Here's how the part is built. I have some questions about the finished solid (model axes, mm). A direction names the side the tool comes from. Round coordinates to 2 decimals unless told otherwise and drop trailing zeros. Loops run counter-clockwise (first coordinate to the right, second up) from the corner with the lowest first, then second, coordinate; pieces in that order, holes last. Notation, with made-up numbers: M -4.5,-27.5 L 17.5,-27.5 A20 cw 17.5,-5.5 Z; hole C 81,82 d5. An arc over 180 degrees is marked long. Put each result on its own line as item: value. Start each with the question number.
```python
from build123d import *

# Parameters (mm, degrees)
SKETCH_3_R           = 9.5
CUT_EXTRUDE_1_DEPTH  = 321.526909947
SKETCH_4_R           = 9.5
CUT_EXTRUDE_2_DEPTH  = 321.526909947
SKETCH_5_R           = 9.5
CUT_EXTRUDE_3_DEPTH  = 321.526909947
SKETCH_6_R           = 9.5
CUT_EXTRUDE_4_DEPTH  = 321.526909947
SKETCH_7_R           = 9.5
CUT_EXTRUDE_5_DEPTH  = 321.526909947
SKETCH_8_R           = 9.5
CUT_EXTRUDE_6_DEPTH  = 321.526909947
SKETCH_9_R           = 9.5
CUT_EXTRUDE_7_DEPTH  = 321.526909947
SKETCH_10_R          = 9.5
CUT_EXTRUDE_8_DEPTH  = 321.526909947
SKETCH_11_R          = 9.5
CUT_EXTRUDE_9_DEPTH  = 321.526909947
SKETCH_12_R          = 9.5
CUT_EXTRUDE_10_DEPTH = 321.526909947
SKETCH_13_R          = 9.5
CUT_EXTRUDE_11_DEPTH = 321.526909947
SKETCH_14_R          = 9.5
CUT_EXTRUDE_12_DEPTH = 321.526909947


with BuildPart() as part:
    # Эскиз1 → Повернуть1 (revolve)
    with BuildSketch(Plane.XY, mode=Mode.PRIVATE) as revolve_1_sk:
        Polygon((0, 0), (265, 0), (265, 127.5), (239, 127.5), (239, 100), (239, 95), (220, 95), (220, 94), (200, 94), (144, 65.5), (70, 65.5), (25, 41), (3, 41), (3, 45), (0, 45), align=None)
    revolve(revolve_1_sk.sketch.rotate(Axis((0, 0, 0), (1, 0, 0)), 90), axis=Axis((0, 0, 0), (1, 0, 0)))

    # Эскиз2 → Вырез-Повернуть1 (revolve, cut)
    with BuildSketch(Plane.XY, mode=Mode.PRIVATE) as cut_revolve_1_sk:
        with BuildLine():
            Line((0, 0), (257, 0))
            Line((257, 0), (257, 34))
            Line((257, 34), (239, 34))
            Line((239, 34), (239, 47))
            Line((239, 47), (220, 47))
            Line((220, 47), (220, 38.502577))
            Line((220, 38.502577), (200, 38.502577))
            Line((200, 38.502577), (200, 55))
            Line((200, 55), (147.669872, 55))
            ThreePointArc((147.669872, 55), (146.273624348, 54.108499061), (146.669872, 52.5))
            Line((146.669872, 52.5), (143.5, 52.5))
            ThreePointArc((143.5, 52.5), (142.75, 52.602347572), (142, 52.5))
            Line((142, 52.5), (90, 52.5))
            ThreePointArc((90, 52.5), (79.13262933, 46.740617582), (70, 38.502577))
            Line((70, 38.502577), (42, 31))
            Line((42, 31), (0, 31))
            Line((0, 31), (0, 0))
        make_face()
    revolve(cut_revolve_1_sk.sketch.rotate(Axis((0, 0, 0), (1, 0, 0)), 90), axis=Axis((0, 0, 0), (1, 0, 0)), mode=Mode.SUBTRACT)

    # Эскиз3 → Вырез-Вытянуть1 (cut, through all)
    with BuildSketch(Plane(origin=(0, 0, 0), x_dir=(0, 0, -1), z_dir=(1, 0, 0))):
        with Locations((0, 113)):
            Circle(SKETCH_3_R)
    extrude(amount=CUT_EXTRUDE_1_DEPTH, mode=Mode.SUBTRACT)

    # Эскиз4 → Вырез-Вытянуть2 (cut, through all)
    with BuildSketch(Plane(origin=(0, 0, 0), x_dir=(0, 0, -1), z_dir=(1, 0, 0))):
        with Locations((-56.5, 97.860870628)):
            Circle(SKETCH_4_R)
    extrude(amount=CUT_EXTRUDE_2_DEPTH, mode=Mode.SUBTRACT)

    # Эскиз5 → Вырез-Вытянуть3 (cut, through all)
    with BuildSketch(Plane(origin=(0, 0, 0), x_dir=(0, 0, -1), z_dir=(1, 0, 0))):
        with Locations((-97.860870628, 56.5)):
            Circle(SKETCH_5_R)
    extrude(amount=CUT_EXTRUDE_3_DEPTH, mode=Mode.SUBTRACT)

    # Эскиз6 → Вырез-Вытянуть4 (cut, through all)
    with BuildSketch(Plane(origin=(0, 0, 0), x_dir=(0, 0, -1), z_dir=(1, 0, 0))):
        with Locations((-113, 0)):
            Circle(SKETCH_6_R)
    extrude(amount=CUT_EXTRUDE_4_DEPTH, mode=Mode.SUBTRACT)

    # Эскиз7 → Вырез-Вытянуть5 (cut, through all)
    with BuildSketch(Plane(origin=(0, 0, 0), x_dir=(0, 0, -1), z_dir=(1, 0, 0))):
        with Locations((-97.860870628, -56.5)):
            Circle(SKETCH_7_R)
    extrude(amount=CUT_EXTRUDE_5_DEPTH, mode=Mode.SUBTRACT)

    # Эскиз8 → Вырез-Вытянуть6 (cut, through all)
    with BuildSketch(Plane(origin=(0, 0, 0), x_dir=(0, 0, -1), z_dir=(1, 0, 0))):
        with Locations((-56.5, -97.860870628)):
            Circle(SKETCH_8_R)
    extrude(amount=CUT_EXTRUDE_6_DEPTH, mode=Mode.SUBTRACT)

    # Эскиз9 → Вырез-Вытянуть7 (cut, through all)
    with BuildSketch(Plane(origin=(0, 0, 0), x_dir=(0, 0, -1), z_dir=(1, 0, 0))):
        with Locations((0, -113)):
            Circle(SKETCH_9_R)
    extrude(amount=CUT_EXTRUDE_7_DEPTH, mode=Mode.SUBTRACT)

    # Эскиз10 → Вырез-Вытянуть8 (cut, through all)
    with BuildSketch(Plane(origin=(0, 0, 0), x_dir=(0, 0, -1), z_dir=(1, 0, 0))):
        with Locations((56.5, -97.860870628)):
            Circle(SKETCH_10_R)
    extrude(amount=CUT_EXTRUDE_8_DEPTH, mode=Mode.SUBTRACT)

    # Эскиз11 → Вырез-Вытянуть9 (cut, through all)
    with BuildSketch(Plane(origin=(0, 0, 0), x_dir=(0, 0, -1), z_dir=(1, 0, 0))):
        with Locations((97.860870628, -56.5)):
            Circle(SKETCH_11_R)
    extrude(amount=CUT_EXTRUDE_9_DEPTH, mode=Mode.SUBTRACT)

    # Эскиз12 → Вырез-Вытянуть10 (cut, through all)
    with BuildSketch(Plane(origin=(0, 0, 0), x_dir=(0, 0, -1), z_dir=(1, 0, 0))):
        with Locations((113, 0)):
            Circle(SKETCH_12_R)
    extrude(amount=CUT_EXTRUDE_10_DEPTH, mode=Mode.SUBTRACT)

    # Эскиз13 → Вырез-Вытянуть11 (cut, through all)
    with BuildSketch(Plane(origin=(0, 0, 0), x_dir=(0, 0, -1), z_dir=(1, 0, 0))):
        with Locations((97.860870628, 56.5)):
            Circle(SKETCH_13_R)
    extrude(amount=CUT_EXTRUDE_11_DEPTH, mode=Mode.SUBTRACT)

    # Эскиз14 → Вырез-Вытянуть12 (cut, through all)
    with BuildSketch(Plane(origin=(0, 0, 0), x_dir=(0, 0, -1), z_dir=(1, 0, 0))):
        with Locations((56.5, 97.860870628)):
            Circle(SKETCH_14_R)
    extrude(amount=CUT_EXTRUDE_12_DEPTH, mode=Mode.SUBTRACT)


solid = part.part
```
1) I'm going to push flat-ended pins straight in: P1, Ø17, axis at y = 56.5, z = -97.86, coming from the -X side; P2, Ø6, axis at x = 233.5, y = -23, coming from the +Z side; P3, Ø3, axis at x = 176, y = -40, coming from the +Z side; P4, Ø24.5, axis at y = 56.5, z = 97.86, coming from the +X side. Where does each tip first touch, or does it pass through?
2) If I drill on probe 1 along Y at (x, z) = (251.75, 0); probe 2 along Z at (x, y) = (255.75, -56.5); probe 3 along Y at (x, z) = (254, -56), over which ranges is the centre line in solid material (lowest first)? Write a range as from..to.
3) On a 3-axis mill with a long thin cutter (end or side, diameter ignored), from which of +Z, -Z, +X, -X, +Y, -Y can I reach the whole of each face in a straight line? I mean faces 5 (the face through (106.482, -19.674, 62.475)), 6 (the face through (251.818, 2.854, 103.939)), 7 (the face through (173.469, 48.794, 25.379)). Say none if no direction works.
4) If we mould it in two halves opening along Z, with no side actions, what happens to faces 1 (the face through (46.47, -9.67, 30.71)), 2 (the face through (251.818, 2.854, -122.061)), 3 (the face through (13.846, 15.703, 37.874)), 4 (the face through (3, 40, 10))? For each: pulls with the +Z half, pulls with the -Z half, needs draft (parallel to the pull), parting line crosses it, or undercut.
5) Suppose I cut it at B-B (z = 0). State how many separate pieces and enclosed holes the cut face has, plus the area to 3 significant figures.
6) Suppose I cut it at A-A (y = 113). Write out the boundary of the cut face in (x, z).
7) Suppose I cut it at D-D (x = 34.5). Write out the boundary of the cut face in (y, z).
Results are:
1. P1: through
1. P2: z = 92.87
1. P3: z = 72.54
1. P4: x = 265
2. probe 1: -127.5..-122.5, -103.5..-34, 34..103.5, 122.5..127.5
2. probe 2: -114.3..-107.36, -88.36..88.36, 107.36..114.3
2. probe 3: -114.54..-107.35, -88.37..88.37, 107.35..114.54
3. face 5: -X
3. face 6: +X, -X
3. face 7: none
4. face 1: undercut
4. face 2: undercut
4. face 3: parting line crosses it
4. face 4: needs draft
5. separate pieces: 3
5. enclosed holes: 0
5. area: 15,700 mm²
6. outline: M 239,-59.05 L 265,-59.05 L 265,-9.5 L 239,-9.5 Z; M 239,9.5 L 265,9.5 L 265,59.05 L 239,59.05 Z
7. outline: C 0,0 d92.34; hole C 0,0 d62
